Input: part model. Units: mm. Frame: model coordinates. Face numbers are marked on the shaded views. A direction names the side the tool comes from. Give positions to 0.01 mm unless a question says otherwise; leave off trailing zeros. Loops run counter-clockwise (first coordinate to the right, second up) from the corner with the lowest first, then second, coordinate; pieces in that order, holes last. Notation, with made-up numbers: M -9,5.5 L 3,5.5 A21 cw 3,19.5 Z; hole C 78,8.5 d9. An arc over 180 degrees is marked long. Return JSON: item names as keys, results as strings. Group by question number.
```python
from build123d import *

# Parameters (mm, degrees)
F0_R     = 13.55
F1_DEPTH = 1.25
F0_R_2   = 12.55
F2_DEPTH = 4.9
F0_R_3   = 1.5
F0_R_4   = 8.5
F3_DEPTH = 1
F0_R_5   = 7.7
F4_DEPTH = 4.9
F5_R     = 7.7
F5_R_2   = 6.2
F6_DEPTH = 2.4


with BuildPart() as f1:
    # F0 (on Front) → F1 (new body)
    with BuildSketch(Plane.XZ):
        Polygon((4.141105, 15.454813), (2.088419, 15.863118), (1.04421, 15.931559), (0, 17.55), (-1.04421, 15.931559), (-2.088419, 15.863118), (-4.141105, 15.454813), (-5.13202, 15.118443), (-6.716094, 16.214086), (-7.061467, 14.319239), (-8, 13.856406), (-9.740183, 12.693653), (-10.526946, 12.003681), (-12.409724, 12.409724), (-12.003681, 10.526946), (-12.693653, 9.740183), (-13.856406, 8), (-14.319239, 7.061467), (-16.214086, 6.716094), (-15.118443, 5.13202), (-15.454813, 4.141105), (-15.863118, 2.088419), (-15.931559, 1.04421), (-17.55, 0), (-15.931559, -1.04421), (-15.863118, -2.088419), (-15.454813, -4.141105), (-15.118443, -5.13202), (-16.214086, -6.716094), (-14.319239, -7.061467), (-13.856406, -8), (-12.693653, -9.740183), (-12.003681, -10.526946), (-12.409724, -12.409724), (-10.526946, -12.003681), (-9.740183, -12.693653), (-8, -13.856406), (-7.061467, -14.319239), (-6.716094, -16.214086), (-5.13202, -15.118443), (-4.141105, -15.454813), (-2.088419, -15.863118), (-1.04421, -15.931559), (0, -17.55), (1.04421, -15.931559), (2.088419, -15.863118), (4.141105, -15.454813), (5.13202, -15.118443), (6.716094, -16.214086), (7.061467, -14.319239), (8, -13.856406), (9.740183, -12.693653), (10.526946, -12.003681), (12.409724, -12.409724), (12.003681, -10.526946), (12.693653, -9.740183), (13.856406, -8), (14.319239, -7.061467), (16.214086, -6.716094), (15.118443, -5.13202), (15.454813, -4.141105), (15.863118, -2.088419), (15.931559, -1.04421), (17.55, 0), (15.931559, 1.04421), (15.863118, 2.088419), (15.454813, 4.141105), (15.118443, 5.13202), (16.214086, 6.716094), (14.319239, 7.061467), (13.856406, 8), (12.693653, 9.740183), (12.003681, 10.526946), (12.409724, 12.409724), (10.526946, 12.003681), (9.740183, 12.693653), (8, 13.856406), (7.061467, 14.319239), (6.716094, 16.214086), (5.13202, 15.118443), align=None)
        Circle(F0_R, mode=Mode.SUBTRACT)
    extrude(amount=F1_DEPTH)

    # F0 (on Front) → F2 (join)
    with BuildSketch(Plane.XZ):
        Circle(F0_R)
        Circle(F0_R_2, mode=Mode.SUBTRACT)
    extrude(amount=F2_DEPTH)

    # F0 (on Front) → F3 (join)
    with BuildSketch(Plane.XZ):
        Circle(F0_R_2)
        with Locations((-2.056837, -10.340419)):
            Circle(F0_R_3, mode=Mode.SUBTRACT)
        with Locations((-10.340419, -2.056837)):
            Circle(F0_R_3, mode=Mode.SUBTRACT)
        with Locations((-5.857377, -8.766184)):
            Circle(F0_R_3, mode=Mode.SUBTRACT)
        with Locations((-8.766184, -5.857377)):
            Circle(F0_R_3, mode=Mode.SUBTRACT)
        with Locations((2.056837, -10.340419)):
            Circle(F0_R_3, mode=Mode.SUBTRACT)
        with Locations((5.857377, -8.766184)):
            Circle(F0_R_3, mode=Mode.SUBTRACT)
        with Locations((8.766184, -5.857377)):
            Circle(F0_R_3, mode=Mode.SUBTRACT)
        with Locations((10.340419, -2.056837)):
            Circle(F0_R_3, mode=Mode.SUBTRACT)
        with Locations((-10.340419, 2.056837)):
            Circle(F0_R_3, mode=Mode.SUBTRACT)
        with Locations((-8.766184, 5.857377)):
            Circle(F0_R_3, mode=Mode.SUBTRACT)
        with Locations((-5.857377, 8.766184)):
            Circle(F0_R_3, mode=Mode.SUBTRACT)
        with Locations((-2.056837, 10.340419)):
            Circle(F0_R_3, mode=Mode.SUBTRACT)
        Circle(F0_R_4, mode=Mode.SUBTRACT)
        with Locations((8.766184, 5.857377)):
            Circle(F0_R_3, mode=Mode.SUBTRACT)
        with Locations((5.857377, 8.766184)):
            Circle(F0_R_3, mode=Mode.SUBTRACT)
        with Locations((10.340419, 2.056837)):
            Circle(F0_R_3, mode=Mode.SUBTRACT)
        with Locations((2.056837, 10.340419)):
            Circle(F0_R_3, mode=Mode.SUBTRACT)
    extrude(amount=F3_DEPTH)

    # F0 (on Front) → F4 (join)
    with BuildSketch(Plane.XZ):
        Circle(F0_R_4)
        Circle(F0_R_5, mode=Mode.SUBTRACT)
    extrude(amount=F4_DEPTH)

    # F5 (on face) → F6 (join)
    with BuildSketch(Plane(origin=(0, 0, 0), x_dir=(-1, 0, 0), z_dir=(0, 1, 0))):
        Circle(F5_R)
        Circle(F5_R_2, mode=Mode.SUBTRACT)
    extrude(amount=-F6_DEPTH)


solid = f1.part
```
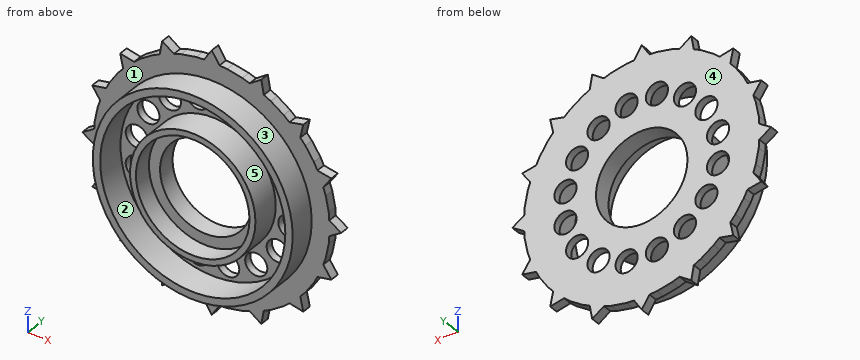
Item 1: Pull-direction query (Z, two-part tool) for the marked faces 1, 2 and 3; classes: pulls with the +Z half, pulls with the -Z half, needs draft (parallel to the pull), parting line crosses it, or undercut.
Item 2: Section B-B, the plane z = 1.5. Give the number of separate pieces and of enclosed holes in the cut face, then the cut area to 3 significant figures.
Item 3: First-contact query: pin 1 Ø2 at (y, z) = (-2, 6) entering from -X; pin 2 Ø1 at (x, y) = (-8, -3.5) entering from -Z; pin 3 Ø8 at (x, z) = (7, -3) entering from +Y; pin 4 Ø2 at (x, y) = (-3, -1.5) entering from -Z. Flat tips, straight axial feed; report the tip coordinate or a pass-through.
Item 4: Section A-A, the plane y = -3.85. Return loops of the section in (x, z).
Item 5: Reachability of the marked faces 4 and 5 from +Z, -Z, +X, -X, +Y, -Y: full face, straight path, thin tool, end or side. Return the list, or none.
Item 6: Material intervals for line 1 (Z direction, x = 0, y = -3.5); line 2 (Z direction, x = -5.5, y = -0.85); line 3 (X direction, y = -4.65, z = -5.5), sorted ascending. Write a range as from..to.
Answer below:
{
 "1": {"face 1": "needs draft", "face 2": "undercut", "face 3": "parting line crosses it"},
 "2": {"separate pieces": "4", "enclosed holes": "0", "area": "33.9 mm^2"},
 "3": {"pin 1": "x = -16.18", "pin 2": "z = -11.29", "pin 3": "y = 0", "pin 4": "z = -15.87"},
 "4": {"outline": "C 0,0 d27.1; C 0,0 d17; hole C 0,0 d25.1; hole C 0,0 d15.4"},
 "5": {"face 4": "+Z, -Z, +X, -X, +Y", "face 5": "-Y"},
 "6": {"line 1": "-13.55..-12.55, -8.5..-7.7, 7.7..8.5, 12.55..13.55", "line 2": "-15.37..-10.22, -7.31..-2.86, 2.86..7.31, 10.22..15.37", "line 3": "-12.38..-11.28, -6.48..-5.39, 5.39..6.48, 11.28..12.38"}
}
